The model under review builds one solid part; all positions refer to its coordinate system, in mm. A direction names the side the tool comes from. Coordinates: 2 decimals unless noted, no trailing zeros. Loops run counter-clockwise (first coordinate to the right, second up) from the corner with the lowest first, then second, coordinate; pieces in that order, holes last. Notation, with made-up numbers: (-23, 16.5) - (31, 16.5) arc R30 ccw to (31, 38.5) - close; hole circle Ø7 at (-18.5, 4.5). An arc over 180 degrees is marked (long way). Use a Markdown table: item, result. Add a question column.
1) Add section A-A, the plane z = 35.5. Give the boundary of the cut face in (x, y), and give its area (3 significant figures).
2) Clearance check with flat-ended pins moving along their axes: pin 1 (10 mm diameter, centred on y = 137.5, z = 46.5, fed in from +X); pin 2 (15 mm diameter, centred on x = 58, z = 20.5, fed in from +Y); pin 3 (24 mm diameter, centred on y = 312, z = 69, fed in from -X); pin 4 (1 mm diameter, centred on x = 43.5, y = 142, fed in from -Z). State where each tip first meets the part, or that it passes through.
3) Add section B-B, the plane x = 92. Give the boundary of the cut face in (y, z).
4) For faces 1 (the flat face through (97.399, 250, 39)), 2 (the flat face through (47, 185, 65)), 3 (the flat face through (59, 0, 39)), 4 (the flat face through (95, 193, 15)), list the 3-axis set-ups (+Z, -Z, +X, -X, +Y, -Y) from which the entire face can be reached by the end or side of a thin tool; tool diameter is ignored.
5) Add section D-D, the plane y = 258.5. Give the boundary of the cut face in (x, z), and give its area (3 significant figures).
6) To check wall thickness, follow L1, parallel to Y at x = 59, z = 69; L2, parallel to Z at x = 65.5, y = 198.5; L3, parallel to Y at x = 72.5, z = 45.5. State the ranges of each line that lie inside material, in increasing order. Write a range as [from, to].
7) Add section C-C, the plane y = 113.5. Give the boundary of the cut face in (x, z).
8) The part is to be moulded in two halves that separate along X. For faces 5 (the flat face through (114.14, 169.84, 66.71)), 6 (the flat face through (86, 298.978, 39)), 7 (the flat face through (95, 317, 15)), 8 (the flat face through (44, 255, 50)), say which applies: pulls with the +X half, pulls with the -X half, needs draft (parallel to the pull), parting line crosses it, or undercut.
```python
from build123d import *

# Parameters (mm, degrees)
EXTRUDE_1_DEPTH     = 80
SKETCH_2_W          = 95
SKETCH_2_H          = 30
CUT_EXTRUDE_1_DEPTH = 150
CUT_EXTRUDE_2_DEPTH = 336


with BuildPart() as part:
    # Эскиз1 → Бобышка-Вытянуть1 (new body)
    with BuildSketch(Plane.XY):
        Polygon((0, 0), (120, 0), (120, 335), (67.160475454, 335), (0, 213.59536065), align=None)
        Polygon((15.034284713, 199.934070047), (69.825157074, 298.978426921), (97.39949173, 298.978426921), (97.39949173, 199.934070047), align=None, mode=Mode.SUBTRACT)
    extrude(amount=EXTRUDE_1_DEPTH)

    # Эскиз2 → Вырез-Вытянуть1 (cut)
    with BuildSketch(Plane(origin=(0, 335, 0), x_dir=(1, 0, 0), z_dir=(0, 1, 0))):
        with Locations((47.5, -15)):
            Rectangle(SKETCH_2_W, SKETCH_2_H)
        with Locations((47.5, -65)):
            Rectangle(SKETCH_2_W, SKETCH_2_H)
    extrude(amount=-CUT_EXTRUDE_1_DEPTH, mode=Mode.SUBTRACT)

    # Эскиз3 → Вырез-Вытянуть2 (cut, through all)
    with BuildSketch(Plane(origin=(0, 335, 0), x_dir=(1, 0, 0), z_dir=(0, 1, 0))):
        Polygon((108.441945131, -10), (108.441945131, -70), (120, -63.32695391), (120, -16.67304609), align=None)
    extrude(amount=-CUT_EXTRUDE_2_DEPTH, mode=Mode.SUBTRACT)


solid = part.part
```
From the geometry:
| question | item | result |
|---|---|---|
| 1 | outline | (0, 0) - (108.44, 0) - (108.44, 335) - (67.16, 335) - (0, 213.6) - close; hole (15.03, 199.93) - (97.4, 199.93) - (97.4, 298.98) - (69.83, 298.98) - close |
| 1 | area | 26,800 mm^2 |
| 2 | pin 1 | stops at x = 108.44 |
| 2 | pin 2 | stops at y = 185 |
| 2 | pin 3 | stops at x = 95 |
| 2 | pin 4 | stops at z = 0 |
| 3 | outline | (0, 0) - (185, 0) - (185, 30) - (199.93, 30) - (199.93, 50) - (185, 50) - (185, 80) - (0, 80) - close; (298.98, 30) - (335, 30) - (335, 50) - (298.98, 50) - close |
| 4 | face 1 | +Z, -Z |
| 4 | face 2 | +Z, -X, +Y |
| 4 | face 3 | +Z, -Z, +X, -X, -Y |
| 4 | face 4 | -Z, -X, +Y |
| 5 | outline | (24.84, 30) - (47.43, 30) - (47.43, 50) - (24.84, 50) - close; (97.4, 0) - (120, 0) - (120, 16.67) - (108.44, 10) - (108.44, 70) - (120, 63.33) - (120, 80) - (97.4, 80) - close |
| 5 | area | 1,640 mm^2 |
| 6 | L1 | y = [0, 185] |
| 6 | L2 | z = [30, 50] |
| 6 | L3 | y = [0, 199.93], [298.98, 335] |
| 7 | outline | (0, 0) - (120, 0) - (120, 16.67) - (108.44, 10) - (108.44, 70) - (120, 63.33) - (120, 80) - (0, 80) - close |
| 8 | face 5 | undercut |
| 8 | face 6 | undercut |
| 8 | face 7 | pulls with the -X half |
| 8 | face 8 | needs draft |
